Geometry: final body of the model. Coordinates: model frame, mm. A direction names the side the tool comes from. Give positions to 0.01 mm unless a question says otherwise; leave off trailing zeros. Write each loop counter-clockwise with the first axis right and the second up, starting at its lowest first coordinate (ties: lowest second). Pieces come first, ordered by that corner, then holes. Notation, with made-up numbers: (75, 44.5) - (129, 44.5) arc R14 ccw to (129, 54.5) - close; hole circle Ø7 at (31.5, 38.5). An arc over 180 degrees is marked (long way). Return JSON: item names as keys, results as strings.
from build123d import *

# Parameters (mm, degrees)
EXTRUDE_1_DEPTH     = 83
CUT_EXTRUDE_1_DEPTH = 26.5
SKETCH_4_R          = 1.45
CUT_EXTRUDE_3_DEPTH = 10
SKETCH_5_R          = 1.45
CUT_EXTRUDE_4_DEPTH = 10
SKETCH_6_R          = 2.65
CUT_EXTRUDE_5_DEPTH = 2
SKETCH_7_R          = 2.8
CUT_EXTRUDE_6_DEPTH = 3


with BuildPart() as part:
    # 草图1 → 凸台-拉伸1 (new body)
    with BuildSketch(Plane.XY):
        Polygon((0, 2.333144796), (0, -50.666855204), (40, 2.333144796), align=None)
    extrude(amount=EXTRUDE_1_DEPTH)

    # 草图3 → 切除-拉伸1 (cut, symmetric)
    with BuildSketch(Plane.XY.offset(41.5)):
        Polygon((36.981132075, -1.666855204), (4.173584906, -1.666855204), (4.173584906, -45.136855204), align=None)
    extrude(amount=CUT_EXTRUDE_1_DEPTH, both=True, mode=Mode.SUBTRACT)

    # 草图4 → 切除-拉伸3 (cut)
    with BuildSketch(Plane(origin=(4.173584906, 0, 0), x_dir=(0, 0, -1), z_dir=(1, 0, 0))):
        with Locations(Location((-31.068580938, -39.636855204, 0), (0, 0, 90))):
            Circle(SKETCH_4_R)
        with Locations(Location((-31.068580938, -28.686855204, 0), (0, 0, 90))):
            Circle(SKETCH_4_R)
        with Locations(Location((-50.38, -28.686855204, 0), (0, 0, 90))):
            Circle(SKETCH_4_R)
        with Locations(Location((-50.38, -39.636855204, 0), (0, 0, 90))):
            Circle(SKETCH_4_R)
    extrude(amount=-CUT_EXTRUDE_3_DEPTH, mode=Mode.SUBTRACT)

    # 草图5 → 切除-拉伸4 (cut)
    with BuildSketch(Plane.XZ.offset(1.666855204)):
        with Locations((13.981132075, 56.5)):
            Circle(SKETCH_5_R)
        with Locations((33.981132075, 56.5)):
            Circle(SKETCH_5_R)
        with Locations((13.981132075, 26.5)):
            Circle(SKETCH_5_R)
        with Locations((33.981132075, 26.5)):
            Circle(SKETCH_5_R)
    extrude(amount=-CUT_EXTRUDE_4_DEPTH, mode=Mode.SUBTRACT)

    # 草图6 → 切除-拉伸5 (cut)
    with BuildSketch(Plane(origin=(4.173584906, 0, 0), x_dir=(0, 0, -1), z_dir=(1, 0, 0))):
        with Locations(Location((-50.38, -28.686855204, 0), (0, 0, 90))):
            Circle(SKETCH_6_R)
        with Locations(Location((-31.068580938, -28.686855204, 0), (0, 0, 90))):
            Circle(SKETCH_6_R)
        with Locations(Location((-50.38, -39.636855204, 0), (0, 0, 90))):
            Circle(SKETCH_6_R)
        with Locations(Location((-31.068580938, -39.636855204, 0), (0, 0, 90))):
            Circle(SKETCH_6_R)
    extrude(amount=-CUT_EXTRUDE_5_DEPTH, mode=Mode.SUBTRACT)

    # 草图7 → 切除-拉伸6 (cut)
    with BuildSketch(Plane.XZ.offset(1.666855204)):
        with Locations((13.981132075, 56.5)):
            Circle(SKETCH_7_R)
        with Locations((33.981132075, 56.5)):
            Circle(SKETCH_7_R)
        with Locations((13.981132075, 26.5)):
            Circle(SKETCH_7_R)
        with Locations((33.981132075, 26.5)):
            Circle(SKETCH_7_R)
    extrude(amount=-CUT_EXTRUDE_6_DEPTH, mode=Mode.SUBTRACT)


solid = part.part
Q1. Mould query, pull axis Z, two halves, no side actions, for faces 4 (the flat face through (15, -18, 0)), 5 (the flat face through (15, 1.333, 55)), 6 (the flat face through (20, 2.333, 41)). Classes: pulls with the +Z half, pulls with the -Z half, needs draft (parallel to the pull), parting line crosses it, or undercut.
Answer key:
{"face 4": "pulls with the -Z half", "face 5": "undercut", "face 6": "needs draft"}
Q2. Section query A-A, the plane z = 50.38. Return the cut outline in (x, y), plus the area to 3 significant figures.
Answer key:
{"outline": "(0, -50.67) - (4.17, -45.14) - (4.17, -42.29) - (2.17, -42.29) - (2.17, -41.09) - (0, -41.09) - close; (0, -38.19) - (2.17, -38.19) - (2.17, -36.99) - (4.17, -36.99) - (4.17, -31.34) - (2.17, -31.34) - (2.17, -30.14) - (0, -30.14) - close; (0, -27.24) - (2.17, -27.24) - (2.17, -26.04) - (4.17, -26.04) - (4.17, -1.67) - (36.98, -1.67) - (40, 2.33) - (0, 2.33) - close", "area": "313 mm^2"}
Q3. Set-up query: faces 1 (the cylindrical face through (3.19, -37.19, 30.05)), 2 (the flat face through (4.174, -23, 42)), 3 (the flat face through (35, 1.333, 25)). Return all of +Z, -Z, +X, -X, +Y, -Y with unobstructed straight access to the full face (end or side cutting, diameter ignored); none if empty.
Answer key:
{"face 1": "+X", "face 2": "+X, -Y", "face 3": "-Y"}
Q4. Section query B-B, the plane x = 14.5. Return the cut outline in (y, z).
Answer key:
{"outline": "(-31.45, 0) - (2.33, 0) - (2.33, 25.15) - (1.33, 25.15) - (1.33, 23.75) - (-1.67, 23.75) - (-1.67, 15) - (-31.45, 15) - close; (-31.45, 68) - (-1.67, 68) - (-1.67, 59.25) - (1.33, 59.25) - (1.33, 57.85) - (2.33, 57.85) - (2.33, 83) - (-31.45, 83) - close; (-1.67, 29.25) - (1.33, 29.25) - (1.33, 27.85) - (2.33, 27.85) - (2.33, 55.15) - (1.33, 55.15) - (1.33, 53.75) - (-1.67, 53.75) - close"}
Q5. Section query C-C, the plane x = 28. Return the cut outline in (y, z).
Answer key:
{"outline": "(-13.57, 0) - (2.33, 0) - (2.33, 83) - (-13.57, 83) - (-13.57, 68) - (-1.67, 68) - (-1.67, 15) - (-13.57, 15) - close"}
Q6. Pin query (flat end, axial travel): P1, Ø6, axis at x = 6.5, z = 9, coming from the -Y side; P2, Ø1.5, axis at y = -10.5, z = 53.5, coming from the +X side; P3, Ø3.5, axis at x = 13.98, z = 56.5, coming from the -Y side; P4, Ø3, axis at y = -26.5, z = 40, coming from the -X side. Return the tip coordinate at first contact, or that it passes through.
Answer key:
{"P1": "stops at y = -46.03", "P2": "stops at x = 4.17", "P3": "stops at y = 1.33", "P4": "stops at x = 0"}
Q7. Material intervals for probe 1 along Y at (x, z) = (3, 50); probe 2 along Z at (x, y) = (26, -8); probe 3 along X at (y, z) = (-16, 57.5), sorted ascending. Write a range as [from, to].
Answer key:
{"probe 1": "y = [-46.69, -42.26], [-37.01, -31.31], [-26.06, 2.33]", "probe 2": "z = [0, 15], [68, 83]", "probe 3": "x = [0, 4.17]"}
Q8. Section query D-D, the plane z = 26.5. Return the cut outline in (x, y).
Answer key:
{"outline": "(0, -50.67) - (4.17, -45.14) - (4.17, -1.67) - (11.18, -1.67) - (11.18, 1.33) - (12.53, 1.33) - (12.53, 2.33) - (0, 2.33) - close; (15.43, 1.33) - (16.78, 1.33) - (16.78, -1.67) - (31.18, -1.67) - (31.18, 1.33) - (32.53, 1.33) - (32.53, 2.33) - (15.43, 2.33) - close; (35.43, 1.33) - (36.78, 1.33) - (36.78, -1.67) - (36.98, -1.67) - (40, 2.33) - (35.43, 2.33) - close"}
